The listing builds one solid part. Answer for the finished solid, in the listing's coordinates (mm). Face numbers are marked on the shaded views. A direction names the side the tool comes from. Coordinates: 2 decimals unless noted, no trailing zeros. Order: outer loops, then holes, each group sorted by start corner. A loop starts at its lowest first (then second) coordinate and runs counter-clockwise, first axis right, second up. Notation, with made-up numbers: (81.25, 75) -> (109.25, 75) arc R25 ccw to (109.25, 93) -> close; hole circle Ø10 at (-33, -14). An arc over 180 degrees is marked (long way). Answer in a Markdown table with one row per item.
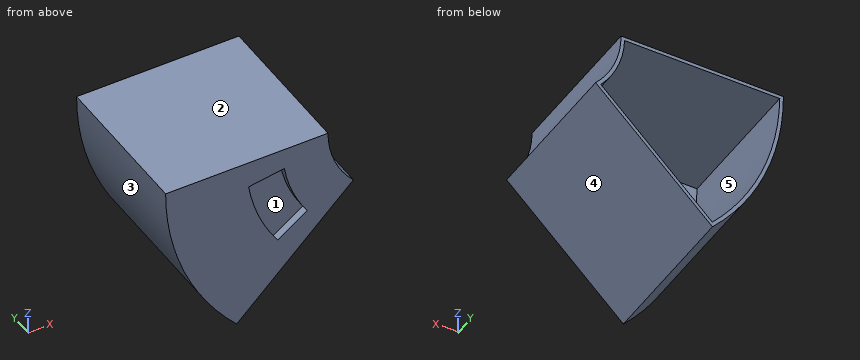
```python
from build123d import *

# Parameters (mm, degrees)
SALIENTE_EXTRUIR1_DEPTH = 40
VACIADO1_T              = -1
SALIENTE_EXTRUIR3_START = 2
SALIENTE_EXTRUIR3_DEPTH = 2
CORTAR_EXTRUIR1_DEPTH   = 2
CROQUIS5_R              = 2.5
CORTAR_EXTRUIR2_DEPTH   = 2


with BuildPart() as part:
    # Croquis1 → Saliente-Extruir1 (new body)
    with BuildSketch(Plane(origin=(0, 0, 0), x_dir=(1, 0, 0), z_dir=(0, 1, 0))):
        with BuildLine():
            Line((-25, 0), (-69.8, 0))
            ThreePointArc((-69.8, 0), (-64.717433049, 26.14754022), (-50.209918064, 48.487154258))
            Line((-50.209918064, 48.487154258), (-17.983495008, 17.366459261))
            ThreePointArc((-17.983495008, 17.366459261), (-23.179596364, 9.365164835), (-25, 0))
        make_face()
    extrude(amount=SALIENTE_EXTRUIR1_DEPTH)

    # Vaciado1
    vaciado1_openings = [part.faces().sort_by_distance(p)[0] for p in [
        (-46.068338787, 40, -18.61281705),
    ]]
    offset(amount=VACIADO1_T, openings=vaciado1_openings, kind=Kind.INTERSECTION)

    # Croquis4 → Saliente-Extruir3 (add)
    with BuildSketch(Plane.XZ.offset(SALIENTE_EXTRUIR3_START)):
        with BuildLine():
            Line((-25, 0), (-69.8, 0))
            ThreePointArc((-69.8, 0), (-64.717433049, -26.14754022), (-50.209918064, -48.487154258))
            Line((-50.209918064, -48.487154258), (-17.983495008, -17.366459261))
            ThreePointArc((-17.983495008, -17.366459261), (-23.179596364, -9.365164835), (-25, 0))
        make_face()
    extrude(amount=-SALIENTE_EXTRUIR3_DEPTH)

    # Croquis2 → Cortar-Extruir1 (cut)
    with BuildSketch(Plane(origin=(0, -2, 0), x_dir=(1, 0, 0), z_dir=(0, 1, 0))):
        with BuildLine():
            Line((-38.909722104, 27.244880727), (-30.718201661, 21.509116363))
            ThreePointArc((-30.718201661, 21.509116363), (-34.769394546, 14.047747253), (-37.038312772, 5.866292439))
            Line((-37.038312772, 5.866292439), (-46.915196178, 7.430637089))
            ThreePointArc((-46.915196178, 7.430637089), (-44.041233092, 17.793813187), (-38.909722104, 27.244880727))
        make_face()
    extrude(amount=CORTAR_EXTRUIR1_DEPTH, mode=Mode.SUBTRACT)

    # Croquis5 → Cortar-Extruir2 (cut)
    with BuildSketch(Plane(origin=(0, 1, 0), x_dir=(1, 0, 0), z_dir=(0, 1, 0))):
        with Locations(Location((-55.631031274, 22.476395605, 0), (0, 0, 270))):
            Circle(CROQUIS5_R)
    extrude(amount=-CORTAR_EXTRUIR2_DEPTH, mode=Mode.SUBTRACT)


solid = part.part
```
(1) A cutting plane is placed at D-D, the plane z = -11. Determine the outline of the cut face in (x, y), then the cut area to 3 significant figures.
Check values:
| item | result |
|---|---|
| outline | (-68.93, -2) -> (-46.21, -2) -> (-46.21, 0) -> (-35.85, 0) -> (-35.85, -2) -> (-22.45, -2) -> (-22.45, 40) -> (-23.56, 40) -> (-23.56, 1) -> (-67.91, 1) -> (-67.91, 40) -> (-68.93, 40) -> close |
| area | 201 mm² |
(2) For a pull along Z with two mould halves and no side action, classify the marked faces 1, 2 and 3 as released by +Z, released by -Z, zero draft, split by the parting line, or undercut.
Check values:
| item | result |
|---|---|
| face 1 | undercut |
| face 2 | released by +Z |
| face 3 | released by -Z |
(3) A cutting plane is placed at A-A, the plane y = 36. Determine the outline of the cut face in (x, z).
Check values:
| item | result |
|---|---|
| outline | (-69.8, 0) arc R69.8 ccw to (-50.21, -48.49) -> (-17.98, -17.37) arc R25 cw to (-25, 0) -> close; hole (-68.79, -1) arc R68.8 ccw to (-50.18, -47.07) -> (-19.38, -17.33) arc R26 cw to (-25.98, -1) -> close |
(4) A cutting plane is placed at B-B, the plane x = -60. Determine the outline of the cut face in (y, z), then the cut area to 3 significant figures.
Check values:
| item | result |
|---|---|
| outline | (-2, -35.67) -> (40, -35.67) -> (40, -33.67) -> (1, -33.67) -> (1, -1) -> (40, -1) -> (40, 0) -> (-2, 0) -> close |
| area | 224 mm² |
(5) Find the intervals of material crossed by line 1 along Y through (x, z) = (-59, -17); line 2 along Z through (x, y) = (-30, 10); line 3 along X through (y, z) = (2, -40), in increasing order. Write a range as from..to.
Check values:
| item | result |
|---|---|
| line 1 | -2..1 |
| line 2 | -28.97..-27.58, -1..0 |
| line 3 | -57.2..-55.98, -42.86..-41.42 |
(6) Which of the six approach directions +Z, -Z, +X, -X, +Y, -Y give full straight-line access (tool end or side, diameter ignored) to the marked faces 4 and 5?
Check values:
| item | result |
|---|---|
| face 4 | -Z, +X, +Y, -Y |
| face 5 | +Y |
(7) A cutting plane is placed at C-C, the plane z = -41. Determine the outline of the cut face in (x, y).
Check values:
| item | result |
|---|---|
| outline | (-56.49, -2) -> (-42.46, -2) -> (-42.46, 40) -> (-43.9, 40) -> (-43.9, 1) -> (-55.25, 1) -> (-55.25, 40) -> (-56.49, 40) -> close |
(8) Flat-ended cylindrical pins translate along their axes: pin 1 (2 mm diameter, centred on x = -44.5, y = 14.5, fed in from -Z); pin 2 (5.5 mm diameter, centred on x = -56, z = -22.5, fed in from +Y); pin 3 (12 mm diameter, centred on x = -40.5, y = 33.5, fed in from -Z). Find the tip coordinate at first contact, or state that the pin passes through.
Check values:
| item | result |
|---|---|
| pin 1 | z = -43.94 |
| pin 2 | y = 1 |
| pin 3 | z = -44.9 |
